Geometry check sheet. Reference: the model listing, model coordinates, mm. Round coordinates to 2 decimals unless told otherwise and drop trailing zeros. Use a Markdown table: item, result. Add a question column.
Q1. Material ranges on L1, parallel to X at y = 10, z = -33.5; L2, parallel to Z at x = 32.5, y = 9.75; L3, parallel to X at y = 9.5, z = -33, recorded low to high.
Q2. Gauge pin test, flat ends, axial feed: P1, Ø3, axis at x = 6.81, z = 11.79, coming from the -Y side; P2, Ø1, axis at y = 11, z = 16, coming from the -X side; P3, Ø2, axis at y = 11.5, z = 32, coming from the -X side; P4, Ø5, axis at x = -20.5, y = 9.5, coming from the -Z side. Record the tip position at first contact, or that the pin passes through.
Q3. Sectioned sample at A-A, the plane x = 0. Give the number of separate pieces and of enclosed holes in the cut face, then the cut area to 3 significant figures.
Autodesk Inventor part; units mm, degrees
ref_plane "YZ Plane" through (0, 0, 0) normal (1, 0, 0) x (0, 1, 0)
ref_plane "XZ Plane" through (0, 0, 0) normal (0, 1, 0) x (-1, 0, 0)
ref_plane "XY Plane" through (0, 0, 0) normal (0, 0, 1) x (1, 0, 0)
sketch "Sketch1" plane through (0, 0, 0) normal (0, 1, 0) x (-1, 0, 0)
  circle A0 centre (0, 0) radius 56.769
  circle A1 centre (0, 0) radius 46.0756
  circle A2 centre (0, 0) radius 31.75
  dimension "d0" = 113.538
  dimension "d1" = 92.1512
  dimension "d2" = 63.5
extrude "Extrusion1" add sketch "Sketch1" along normal blind 17.272 contours A0 | A1 | A2
sketch "Sketch2" plane through (0, 17.272, 0) normal (0, 1, 0) x (1, 0, 0)
  circle A0 centre (0, 0) radius 46.0756
  circle A1 centre (-46.0756, 0) radius 4.0894
  dimension "d5" = 92.1512
  dimension "d6" = 8.1788
hole "Hole1" at (-46.0756, 17.272, 0) direction (0, -1, 0) diameter 8.4328 end through all
pattern_circular "Circular Pattern1" count 8 over 360 about axis through (0, 0, 0) along (0, 1, 0) of "Hole1"
sketch "Sketch4" plane through (0, 17.272, 0) normal (0, 1, 0) x (1, 0, 0)
  circle A0 centre (0, 0) radius 14.7993
hole "Hole2" at (0, 17.272, 0) direction (0, -1, 0) diameter 63.5 end through all
sketch "Sketch6" plane through (0, 0, 0) normal (0, 1, 0) x (-1, 0, 0)
  circle A0 centre (0, 0) radius 31.75
  circle A1 centre (0, 0) radius 19.05
extrude "Extrusion3" add sketch "Sketch6" along normal blind 17.272
sketch "Sketch7" plane through (0, 17.272, 0) normal (0, 1, 0) x (1, 0, 0)
  circle A0 centre (0, 0) radius 34.29
  circle A1 centre (0, 0) radius 31.75
  circle A2 centre (0, 0) radius 25.4
  circle A3 centre (0, 0) radius 27.94
  dimension "d35" = 68.58
  dimension "d36" = 63.5
  dimension "d37" = 50.8
  dimension "d38" = 55.88
extrude "Extrusion4" cut sketch "Sketch7" against normal blind 1.27 contours A0
sketch "Sketch9" plane through (0, 17.272, 0) normal (0, 1, 0) x (1, 0, 0)
  circle A0 centre (0, 0) radius 27.94
  circle A1 centre (0, 0) radius 31.75
  dimension "d45" = 55.88
  dimension "d46" = 63.5
extrude "Extrusion6" cut sketch "Sketch9" against normal blind 2.54
chamfer "Chamfer1" distance 0.254 angle 45 1 edges at (-46.0756, 17.272, -4.2164)
chamfer "Chamfer2" distance 0.254 angle 45 1 edges at (-46.0756, 0, -4.2164)
chamfer "Chamfer3" distance 0.762 angle 45 2 edges at (56.769, 17.272, 0) (56.769, 0, 0)
sketch "Sketch10" plane through (0, 17.272, 0) normal (0, 1, 0) x (1, 0, 0)
  circle A0 centre (32.5804, 32.5804) radius 4.2164
  circle A1 centre (46.0756, 0) radius 4.2164
  line L0 (32.5804, 32.5804) -> (46.0756, 0)
  line L1 (46.0756, 0) -> (39.328, 16.2902)
  circle A2 centre (-46.0756, 0) radius 4.4704
  circle A3 centre (-32.5804, -32.5804) radius 4.2164
  line L2 (-46.0756, 0) -> (-32.5804, -32.5804)
  line L3 (39.328, 16.2902) -> (-39.328, -16.2902)
  line L4 (-39.328, -16.2902) -> (52.9444, 21.9303)
  line L5 (-39.328, -16.2902) -> (60.5469, -16.2902) construction
  line L6 (52.9444, 21.9303) -> (-52.9809, -21.9454)
  line L7 (39.328, 16.2902) -> (39.6342, 15.551)
  line L8 (39.6342, 15.551) -> (39.0218, 17.0294)
  line L9 (39.0218, 17.0294) -> (52.0886, 22.4418)
  line L10 (39.0218, 17.0294) -> (53.1652, 17.0294) construction
  line L11 (52.0886, 22.4418) -> (31.2876, 13.8258)
  line L12 (39.6342, 15.551) -> (52.7487, 20.9832)
  circle A4 centre (0, 0) radius 56.769
  line L13 (39.6342, 15.551) -> (53.8292, 15.551) construction
  line L14 (52.7487, 20.9832) -> (52.7487, 20.9832)
  line L15 (52.7487, 20.9832) -> (31.9774, 12.3794)
  circle A5 centre (0, 0) radius 34.29
  line L16 (31.2876, 13.8258) -> (52.0886, 22.4418)
  line L17 (52.0886, 22.4418) -> (52.7487, 20.9832)
  line L18 (52.0886, 22.4418) -> (31.2876, 13.8258)
  point P0 (31.365, 13.8578)
  dimension "d58" = 22.5
  dimension "d59" = 0.8001
  dimension "d60" = 1.6002
  dimension "d61" = 22.5
  dimension "d62" = 22.5
extrude "Extrusion7" cut sketch "Sketch10" against normal blind 1.016 contours L9 L17 L4 L0 | L0 L3 A5 L11 | L4 L17 L12 L0 | L0 L15 A5 L3
sketch "Sketch11" plane through (0, 17.272, 0) normal (0, 1, 0) x (1, 0, 0)
  line L0 (31.365, 13.8578) -> (51.4323, 22.17)
  line L1 (52.0446, 20.6916) -> (31.9774, 12.3794)
  line L2 (51.4323, 22.17) -> (31.365, 13.8578)
  line L3 (31.365, 13.8578) -> (-52.6609, -20.9468)
  line L4 (52.0446, 20.6916) -> (31.9774, 12.3794)
  circle A0 centre (0, 0) radius 56.769
  line L5 (-52.1363, -22.4616) -> (31.9774, 12.3794)
  line L6 (-52.1363, -22.4616) -> (-52.6609, -20.9468)
  arc A1 (31.365, 13.8578) -> (31.9774, 12.3794) centre (0, 0) ccw
  circle A2 centre (0, 0) radius 34.29
  line L7 (-31.365, -13.8578) -> (-31.9774, -12.3794)
  point P0 (-31.365, -13.8578)
extrude "Extrusion8" cut sketch "Sketch11" against normal blind 1.016 contours A1 L5 L6 L3
sketch "Sketch13" plane through (0, 0, 0) normal (0, -1, 0) x (1, 0, 0)
  circle A0 centre (0, 0) radius 27.94
  circle A1 centre (0, 0) radius 31.75
  circle A2 centre (0, 0) radius 34.29
extrude "Extrusion9" cut sketch "Sketch13" against normal blind 2.54 contours A1
extrude "Extrusion10" cut sketch "Sketch13" against normal blind 1.27 contours A2
sketch "Sketch14" plane through (0, 0, 0) normal (0, -1, 0) x (1, 0, 0)
  line L0 (31.365, -13.8578) -> (52.0886, -22.4418)
  line L1 (52.7487, -20.9832) -> (31.9774, -12.3794)
  line L2 (-52.6609, 20.9468) -> (-31.9774, 12.3794)
  line L3 (-31.365, 13.8578) -> (-52.1363, 22.4616)
  line L4 (51.4323, -22.17) -> (52.0886, -22.4418)
  line L5 (52.0886, -22.4418) -> (31.365, -13.8578)
  arc A0 (52.7487, -20.9832) -> (-52.1363, 22.4616) centre (0, 0) ccw
  line L6 (31.9774, -12.3794) -> (52.7487, -20.9832)
  line L7 (52.7487, -20.9832) -> (52.0886, -22.4418)
  circle A1 centre (0, 0) radius 34.29
  line L8 (-31.9774, 12.3794) -> (-31.365, 13.8578)
  circle A2 centre (0, 0) radius 56.769
  line L9 (-52.1363, 22.4616) -> (-52.6609, 20.9468)
extrude "Extrusion11" cut sketch "Sketch14" against normal blind 1.016 contours A1 L1 L7 L0
extrude "Extrusion12" cut sketch "Sketch14" against normal blind 1.016 contours L2 L9 L3 A1
sketch "Sketch15" plane through (0, 0, 0) normal (0, 1, 0) x (-1, 0, 0)
  circle A0 centre (0, 0) radius 19.05
extrude "Extrusion13" add sketch "Sketch15" along normal blind 17.272
sketch "Sketch17" plane through (0, 0, 0) normal (0, -1, 0) x (1, 0, 0)
  circle A0 centre (0, 0) radius 27.94
hole "Hole4" at (0, 0, 0) direction (0, 1, 0) diameter 6.35 end through all
sketch "Sketch18" plane through (0, 0, 0) normal (0, -1, 0) x (1, 0, 0)
  line L0 (0, 0) -> (-13.6144, 0)
  dimension "d103" = 13.6144
hole "Hole5" at (-13.6144, 0, 0) direction (0, 1, 0) diameter 4.9022 end through all
pattern_circular "Circular Pattern5" count 3 over 360 about axis through (0, 161.4933, 0) along (0, -1, 0) of "Hole5"
properties part number "4.5 flange"
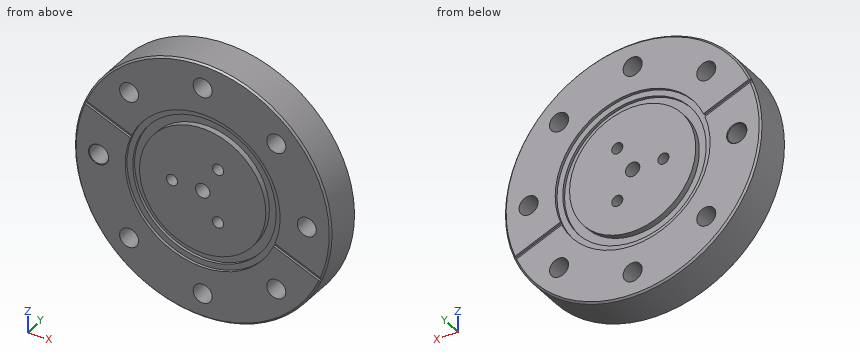
Values:
| question | item | result |
|---|---|---|
| 1 | L1 | -45.83 to -36.7, -28.47 to 28.47, 36.7 to 45.83 |
| 1 | L2 | -46.55 to -36.8, -28.36 to 28.36, 36.8 to 46.55 |
| 1 | L3 | -46.19 to -36.78, -28.38 to 28.38, 36.78 to 46.19 |
| 2 | P1 | through |
| 2 | P2 | x = -54.61 |
| 2 | P3 | x = -47.56 |
| 2 | P4 | z = -53.84 |
| 3 | separate pieces | 4 |
| 3 | enclosed holes | 0 |
| 3 | area | 1,510 mm^2 |
